from build123d import *

# Parameters (mm, degrees)
F0_R      = 30.1625
F1_DEPTH  = 0.9652
F2_W      = 76.2
F2_H      = 76.2
F2_W_2    = 57.785
F2_H_2    = 57.785
F3_DEPTH  = 0.9662
F4_R      = 1.905
F5_DEPTH  = 1.5748
F6_R      = 1.905
F7_DEPTH  = 1.5748
F9_DEPTH  = 25.4
F11_DEPTH = 25.4
F13_DEPTH = 10.922


with BuildPart() as f1:
    # F0 (on Top) → F1 (new body)
    with BuildSketch(Plane.XY):
        Circle(F0_R)
    extrude(amount=F1_DEPTH)

    # F2 (on Top) → F3 (cut, through all)
    with BuildSketch(Plane.XY):
        Rectangle(F2_W, F2_H)
        Rectangle(F2_W_2, F2_H_2, mode=Mode.SUBTRACT)
    extrude(amount=F3_DEPTH, mode=Mode.SUBTRACT)

    # F4 (on face) → F5 (join)
    with BuildSketch(Plane.XY.offset(0.9652)):
        with Locations((-9.332556, 5.388154)):
            Circle(F4_R)
        with Locations((5.388154, 9.332556)):
            Circle(F4_R)
        with Locations((9.332556, -5.388154)):
            Circle(F4_R)
        with Locations((-5.388154, -9.332556)):
            Circle(F4_R)
    extrude(amount=F5_DEPTH)

    # F6 (on face) → F7 (join)
    with BuildSketch(Plane.XY.offset(0.9652)):
        with Locations((6.245304, 23.30779)):
            Circle(F6_R)
        with Locations((-16.749408, 17.369924)):
            Circle(F6_R)
        with Locations((-6.245304, -23.30779)):
            Circle(F6_R)
        with Locations((16.749408, -17.369924)):
            Circle(F6_R)
        with Locations((21.869207, 10.197779)):
            Circle(F6_R)
        with Locations((-21.869207, -10.197779)):
            Circle(F6_R)
    extrude(amount=F7_DEPTH)

    # F8 (on face) → F9 (cut)
    with BuildSketch(Plane.XY.offset(0.9652)):
        Polygon((11.396703, -25.19386), (12.548755, -27.457568), (14.812463, -26.305517), (13.660412, -24.041808), align=None)
    extrude(amount=-F9_DEPTH, mode=Mode.SUBTRACT)

    # F10 (on face) → F11 (cut)
    with BuildSketch(Plane.XY.offset(0.9652)):
        Polygon((-10.851198, 28.321521), (-16.510447, 25.441348), (-12.363614, 17.29324), (-6.704365, 20.173413), align=None)
    extrude(amount=-F11_DEPTH, mode=Mode.SUBTRACT)

    # F12 (on face) → F13 (join)
    with BuildSketch(Plane(origin=(0, 0, 0), x_dir=(1, 0, 0), z_dir=(0, 0, -1))):
        Polygon((-28.784711, -3.94695), (13.750207, -25.594331), (28.784711, 3.94695), (-13.750207, 25.594331), align=None)
    extrude(amount=F13_DEPTH)


solid = f1.part
Check sheet for the modelled part. Datum: model origin and axes. Units: mm. A direction names the side the tool comes from. Give positions to 0.01 mm unless a question says otherwise; leave off trailing zeros. Write each loop counter-clockwise with the first axis right and the second up, starting at its lowest first coordinate (ties: lowest second). Pieces come first, ordered by that corner, then holes. Notation, with made-up numbers: (36, -30.5) -> (82, -30.5) arc R10 cw to (82, -15.5) -> close; hole circle Ø4 at (-36.75, -19). An arc over 180 degrees is marked (long way). Use one line per item in the form item = value. Start each with the question number.
1. Go/stop test with flat-tipped pins: P1, Ø1, axis at x = 14.5, y = -21.5, coming from the -Z side; P2, Ø3, axis at x = 10, z = -3.5, coming from the -Y side; P3, Ø1.5, axis at x = 22.5, y = 7, coming from the +Z side. Record where each tip stops, or that it passes through.
2. Section check B-B (x = 6). Record the cut outline in (y, z).
3. Access from +Z, -Z, +X, -X, +Y, -Y to the whole of each face (thin tool, end or side, straight path). Record for faces 4 (the flat face through (-7.81, 14.62, -5.38)), 5 (the flat face through (7.81, -14.62, -5.38)), 6 (the cylindrical face through (4.342, 23.392, 1.742)).
4. Thickness scan on line 1 along Z through (x, y) = (-7, -14); line 2 along Z through (x, y) = (-16, 12.5); line 3 along Y through (x, z) = (-6.5, -4.5). Record the ranges inside material, lowest first. Write a range as from..to.
5. Section check D-D (y = -16.5). Record the cut outline in (x, z).
6. Section check A-A (y = -6.5). Record the cut outline in (x, z).
7. Mould release check, pull along X, two halves, no side actions. Record for faces 1 (the cylindrical face through (3.485, 9.416, 1.742)), 2 (the flat face through (8, -15, 0)), 3 (the cylindrical face through (10.6, -28.24, 0.48)): pulls with the +X half, pulls with the -X half, needs draft (parallel to the pull), parting line crosses it, or undercut.
8. Section check C-C (z = -6). Record the cut outline in (x, y), and give its area (3 significant figures).
Conclusion:
q1.P1 = 0
q1.P2 = -14.27
q1.P3 = 0.97
q2.outline = (-28.89, 0) -> (-15.54, 0) -> (-15.54, -10.92) -> (21.65, -10.92) -> (21.65, 0) -> (28.89, 0) -> (28.89, 0.97) -> (25.2, 0.97) -> (25.2, 2.54) -> (21.42, 2.54) -> (21.42, 0.97) -> (11.14, 0.97) -> (11.14, 2.54) -> (7.53, 2.54) -> (7.53, 0.97) -> (-28.89, 0.97) -> close
q3.face_4 = -Z, -X, +Y
q3.face_5 = -Z, +X, -Y
q3.face_6 = +Z
q4.line_1 = -10.92..0.97
q4.line_2 = 0..0.97
q4.line_3 = -21.9..15.29
q5.outline = (-25.25, 0) -> (-18.38, 0) -> (-18.38, -10.92) -> (4.12, -10.92) -> (4.12, 0) -> (25.25, 0) -> (25.25, 0.97) -> (18.44, 0.97) -> (18.44, 2.54) -> (15.05, 2.54) -> (15.05, 0.97) -> (-25.25, 0.97) -> close
q6.outline = (-28.89, 0) -> (-23.47, 0) -> (-23.47, -10.92) -> (23.77, -10.92) -> (23.77, 0) -> (28.89, 0) -> (28.89, 0.97) -> (10.88, 0.97) -> (10.88, 2.54) -> (7.79, 2.54) -> (7.79, 0.97) -> (-28.89, 0.97) -> close
q7.face_1 = undercut
q7.face_2 = needs draft
q7.face_3 = pulls with the +X half
q8.outline = (-28.78, 3.95) -> (-13.75, -25.59) -> (28.78, -3.95) -> (13.75, 25.59) -> close
q8.area = 1,580 mm²
